The model under review builds one solid part; all positions refer to its coordinate system, in mm. Give positions to 0.01 mm unless a question says otherwise; leave off trailing zeros. Order: outer loops, then holes, each group sorted by start corner. A loop starts at its lowest first (then second) coordinate and runs counter-clockwise, first axis right, second up. Notation, with made-up numbers: (14.5, 0) - (46.5, 0) arc R34 cw to (46.5, 34) - close; hole circle Ø10 at (11.5, -14.75). An arc over 180 degrees is marked (long way). Use CSV: the item, a comma, the result in double quotes. Start each with the question number.
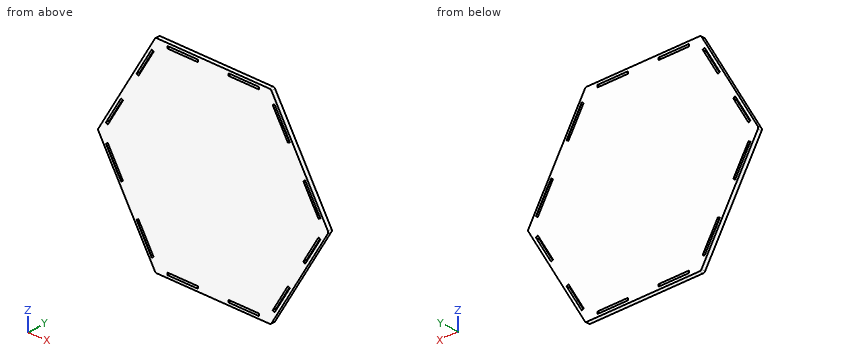
```python
from build123d import *

# Parameters (mm, degrees)
F1_DEPTH        = 5.08
F2_W            = 38.4310525078
F2_H            = 2.7686
F3_DEPTH        = 5.08
F3_COPIES_COUNT = 6


# Not quite as in the source:
# - a pattern or mirror of a feature is missing from the dataset's text; its kind, count and spacing are read off the source's solid


with BuildPart() as f1:
    # F0 (on Front) → F1 (new body)
    with BuildSketch(Plane.XZ):
        with BuildLine():
            Line((71.1237796615, 125.73), (-71.1237796615, 125.73))
            ThreePointArc((-71.1237796615, 125.73), (-72.3937796615, 125.3897045256), (-73.3234841871, 124.46))
            Line((-73.3234841871, 124.46), (-144.4472638486, 1.27))
            ThreePointArc((-144.4472638486, 1.27), (-144.7875593229, 0), (-144.4472638486, -1.27))
            Line((-144.4472638486, -1.27), (-73.3234841871, -124.46))
            ThreePointArc((-73.3234841871, -124.46), (-72.3937796615, -125.3897045256), (-71.1237796615, -125.73))
            Line((-71.1237796615, -125.73), (71.1237796615, -125.73))
            ThreePointArc((71.1237796615, -125.73), (72.3937796615, -125.3897045256), (73.3234841871, -124.46))
            Line((73.3234841871, -124.46), (144.4472638486, -1.27))
            ThreePointArc((144.4472638486, -1.27), (144.7875593229, 0), (144.4472638486, 1.27))
            Line((144.4472638486, 1.27), (73.3234841871, 124.46))
            ThreePointArc((73.3234841871, 124.46), (72.3937796615, 125.3897045256), (71.1237796615, 125.73))
        make_face()
    extrude(amount=F1_DEPTH)

    # F2 (on face) → F3 (cut, through all)
    with BuildSketch(Plane.XZ.offset(5.08)):
        with Locations((-38.5195262539, 121.1707)):
            Rectangle(F2_W, F2_H)
        with Locations((38.5195262539, 121.1707)):
            Rectangle(F2_W, F2_H)
    f3 = extrude(amount=-F3_DEPTH, mode=Mode.SUBTRACT)

    # F3_copies: F3 ×6 about axis
    f3_copies_axis = Axis((0, 0, 0), (0, 1, 0))
    for i in range(1, F3_COPIES_COUNT):
        add(f3.rotate(f3_copies_axis, i * 360 / F3_COPIES_COUNT), mode=Mode.SUBTRACT)


solid = f1.part
```
1. Clearance check with flat-ended pins moving along their axes: pin 1 (1 mm diameter, centred on y = -1, z = 29.5, fed in from +X); pin 2 (1 mm diameter, centred on y = -1, z = -83.5, fed in from +X); pin 3 (3 mm diameter, centred on y = -2, z = 121, fed in from +X); pin 4 (8 mm diameter, centred on x = -81, z = 39.5, fed in from +Y). State where each tip first meets the part, or that it passes through.
2. Consider section A-A (x = 51). Give the boundary of the cut face in (y, z) (3 decimals), and give its area (3 significant figures).
3. Consider section C-C (y = -3.9). State how many separate pieces and enclosed holes the cut face has, and give its area (3 significant figures).
4. To check wall thickness, follow L1, parallel to Z at x = 39, y = -3.65 (3 decimals); L2, parallel to Z at x = 78, y = -0.9; L3, parallel to X at y = -0.95, z = -18. State the ranges of each line that lie inside material, in increasing order. Write a range as [from, to].
5. Consider section D-D (z = -55). Give the boundary of the cut face in (x, y), and give its area (3 significant figures).
6. Consider section B-B (z = 83.5). Give the boundary of the cut face in (x, y), and give its area (3 significant figures).
Answers follow:
1,pin 1,"stops at x = 128.44"
1,pin 2,"stops at x = 97.26"
1,pin 3,"stops at x = 76.19"
1,pin 4,"stops at y = 0"
2,outline,"(-5.08, -125.73) - (0, -125.73) - (0, -122.555) - (-5.08, -122.555) - close; (-5.08, -119.786) - (0, -119.786) - (0, 119.786) - (-5.08, 119.786) - close; (-5.08, 122.555) - (0, 122.555) - (0, 125.73) - (-5.08, 125.73) - close"
2,area,"1,250 mm^2"
3,separate pieces,"1"
3,enclosed holes,"12"
3,area,"53,500 mm^2"
4,L1,"z = [-125.73, -122.555], [-119.786, 119.786], [122.555, 125.73]"
4,L2,"z = [-116.36, -110.01], [-104.47, 104.47], [110.01, 116.36]"
4,L3,"x = [-134.79, -131.12], [-127.93, 127.93], [131.12, 134.79]"
5,outline,"(-113.43, -5.08) - (113.43, -5.08) - (113.43, 0) - (-113.43, 0) - close"
5,area,"1,150 mm^2"
6,outline,"(-96.97, -5.08) - (-93.31, -5.08) - (-93.31, 0) - (-96.97, 0) - close; (-90.11, -5.08) - (90.11, -5.08) - (90.11, 0) - (-90.11, 0) - close; (93.31, -5.08) - (96.97, -5.08) - (96.97, 0) - (93.31, 0) - close"
6,area,"953 mm^2"
